```python
from build123d import *

# Parameters (mm, degrees)
SKETCH1_R           = 38.1
BOSS_EXTRUDE1_DEPTH = 10.16
SKETCH2_W           = 31.75
SKETCH2_H           = 31.75
BOSS_EXTRUDE3_DEPTH = 31.75
SKETCH3_W           = 25.4
SKETCH3_H           = 25.4
CUT_EXTRUDE1_DEPTH  = 42.91
SKETCH4_R           = 3.175
CUT_EXTRUDE2_DEPTH  = 54.975


with BuildPart() as part:
    # Sketch1 → Boss-Extrude1 (new body)
    with BuildSketch(Plane(origin=(0, 0, 0), x_dir=(1, 0, 0), z_dir=(0, 1, 0))):
        Circle(SKETCH1_R)
    extrude(amount=BOSS_EXTRUDE1_DEPTH)

    # Sketch2 → Boss-Extrude3 (add)
    with BuildSketch(Plane(origin=(0, 10.16, 0), x_dir=(1, 0, 0), z_dir=(0, 1, 0))):
        Rectangle(SKETCH2_W, SKETCH2_H)
    extrude(amount=BOSS_EXTRUDE3_DEPTH)

    # Sketch3 → Cut-Extrude1 (cut, through all)
    with BuildSketch(Plane(origin=(0, 41.91, 0), x_dir=(1, 0, 0), z_dir=(0, 1, 0))):
        Rectangle(SKETCH3_W, SKETCH3_H)
    extrude(amount=-CUT_EXTRUDE1_DEPTH, mode=Mode.SUBTRACT)

    # Sketch4 → Cut-Extrude2 (cut, through all)
    with BuildSketch(Plane.XY.offset(15.875)):
        with Locations((0, 32.385)):
            Circle(SKETCH4_R)
    extrude(amount=-CUT_EXTRUDE2_DEPTH, mode=Mode.SUBTRACT)


solid = part.part
```
For this review, take the finished solid that the model builds, in its own axes (mm). A direction names the side the tool comes from. Round coordinates to 2 decimals unless told otherwise and drop trailing zeros. Write each loop counter-clockwise with the first axis right and the second up, starting at its lowest first coordinate (ties: lowest second). Pieces come first, ordered by that corner, then holes. Notation, with made-up numbers: (-7, 72.5) - (1, 72.5) arc R23 cw to (1, 93.5) - close; hole circle Ø2 at (-32.75, -25.75). An arc over 180 degrees is marked (long way). Answer as a JSON object with one key per item and string values.
1. Tool access review of faces 5 (the face through (0, 21, 12.7)), 6 (the face through (16.4, 10.16, -0.5)), 7 (the face through (0, 26, 15.875)), 8 (the face through (0, 26, -15.875)), 9 (the face through (1.71, 35.06, -14.27)): name each direction out of +Z, -Z, +X, -X, +Y, -Y from which nothing blocks a thin tool from reaching the whole face with its end or side.
Response values:
{"face 5": "+Y, -Y", "face 6": "+Y", "face 7": "+Z, +X, -X, +Y", "face 8": "-Z, +X, -X, +Y", "face 9": "+Z, -Z"}
2. For pin 1 Ø12.5 at (x, y) = (1, 16.5) entering from +Z (3 decimals); pin 2 Ø16 at (y, z) = (19, 7.5) entering from -X (3 decimals); pin 3 Ø2 at (x, y) = (8, 9.5) entering from -Z; pin 4 Ø5 at (x, y) = (0, 32.385) entering from -Z, all flat-tipped, find the tip position at first contact; note any pin that passes through.
Response values:
{"pin 1": "stops at z = 15.875", "pin 2": "stops at x = -15.875", "pin 3": "stops at z = -37.45", "pin 4": "passes through"}
3. To check wall thickness, follow line 1 along Z through (x, y) = (-12, 33) (3 decimals); line 2 along Y through (x, z) = (0, -14); line 3 along Y through (x, z) = (1.5, -28.5). State the ranges of each line that lie inside material, in increasing order.
Response values:
{"line 1": "z = -15.875 to -12.7, 12.7 to 15.875", "line 2": "y = 0 to 29.21, 35.56 to 41.91", "line 3": "y = 0 to 10.16"}
4. We need section A-A on z = 0. Give the boundary of the cut face in (x, y) (3 decimals), then the cut area to 3 significant figures.
Response values:
{"outline": "(-38.1, 0) - (-12.7, 0) - (-12.7, 41.91) - (-15.875, 41.91) - (-15.875, 10.16) - (-38.1, 10.16) - close; (12.7, 0) - (38.1, 0) - (38.1, 10.16) - (15.875, 10.16) - (15.875, 41.91) - (12.7, 41.91) - close", "area": "718 mm2"}
5. Draft analysis for pull direction X (two halves, no side actions). For faces 1 (the face through (-15.875, 26, 0)), 2 (the face through (-12.7, 21, 0)), 3 (the face through (15.875, 26, 0)), 4 (the face through (-30.235, 5.009, 23.183)), state which applies: +X half, -X half, draft (parallel to the pull), parting line (faces both ways), or undercut.
Response values:
{"face 1": "-X half", "face 2": "undercut", "face 3": "+X half", "face 4": "parting line"}
6. We need section C-C on x = 0. Give the boundary of the cut face in (y, z) (3 decimals).
Response values:
{"outline": "(0, -38.1) - (10.16, -38.1) - (10.16, -15.875) - (29.21, -15.875) - (29.21, -12.7) - (0, -12.7) - close; (0, 12.7) - (29.21, 12.7) - (29.21, 15.875) - (10.16, 15.875) - (10.16, 38.1) - (0, 38.1) - close; (35.56, -15.875) - (41.91, -15.875) - (41.91, -12.7) - (35.56, -12.7) - close; (35.56, 12.7) - (41.91, 12.7) - (41.91, 15.875) - (35.56, 15.875) - close"}
7. We need section B-B on y = 13.5. Give the boundary of the cut face in (x, z) (3 decimals), then the cut area to 3 significant figures.
Response values:
{"outline": "(-15.875, -15.875) - (15.875, -15.875) - (15.875, 15.875) - (-15.875, 15.875) - close; hole (-12.7, -12.7) - (12.7, -12.7) - (12.7, 12.7) - (-12.7, 12.7) - close", "area": "363 mm2"}
8. We need section D-D on x = 9. Give the boundary of the cut face in (y, z) (3 decimals).
Response values:
{"outline": "(0, -37.022) - (10.16, -37.022) - (10.16, -15.875) - (41.91, -15.875) - (41.91, -12.7) - (0, -12.7) - close; (0, 12.7) - (41.91, 12.7) - (41.91, 15.875) - (10.16, 15.875) - (10.16, 37.022) - (0, 37.022) - close"}
